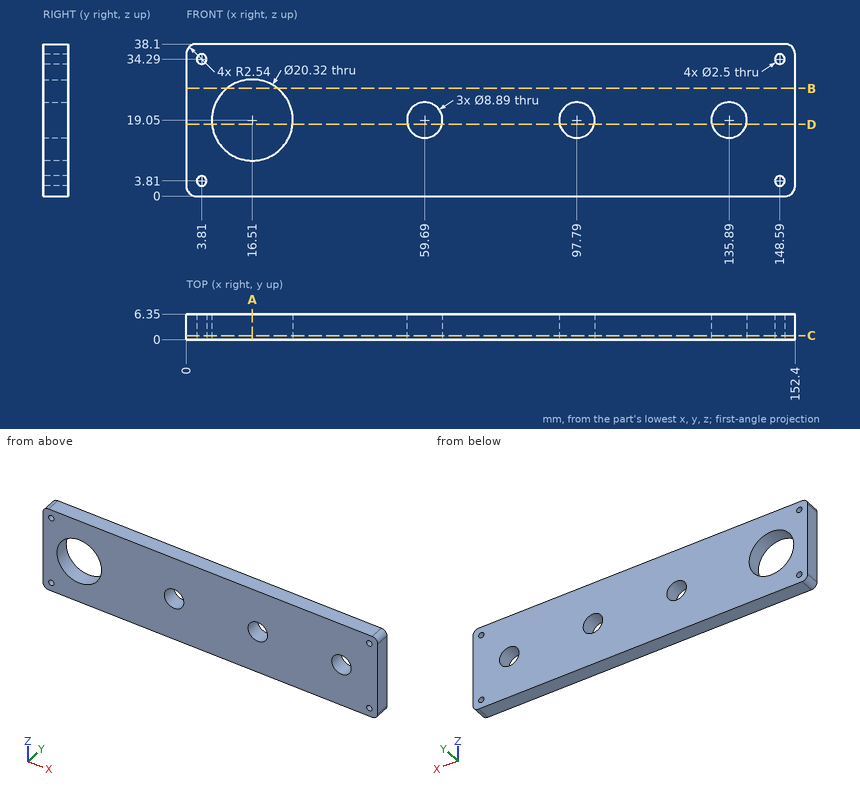
Could you check a few things on this drawing? It's one solid part, dimensions in mm from its lowest x, y, z. Coordinates: 2 decimals unless noted, no trailing zeros. Order: outer loops, then holes, each group sorted by start corner. A loop starts at its lowest first (then second) coordinate and runs counter-clockwise, first axis right, second up. Notation, with made-up numbers: M 17.5,80 L 68.5,80 A15 cw 68.5,95 Z; hole C -9,15 d11. An arc over 180 degrees is marked long. Answer as a JSON object with one key per item and string values. Group by question number.
(1) I need wall thicknesses on probe 1 along Z at (x, y) = (3.81, 3.5); probe 2 along X at (y, z) = (3.5, 19.05) (3 decimals); probe 3 along Z at (x, y) = (59.69, 4.5) (3 decimals). Which ranges of each line are inside material? Lowest first, please.
(2) Suppose I cut it at C-C, the plane y = 1. State how many separate pieces and enclosed holes the cut face has, then the cut area to 3 significant figures.
(3) Suppose I cut it at B-B, the plane z = 27. Please give me the cut outline in (x, y), then the cut area to 3 significant figures.
(4) Suppose I cut it at D-D, the plane z = 18. Please give me the cut outline in (x, y).
(5) Suppose I cut it at A-A, the plane x = 16.51. Please give me the cut outline in (y, z).
Values found:
{
 "1": {"probe 1": "z = 0 to 2.56, 5.06 to 33.04, 35.54 to 38.1", "probe 2": "x = 0 to 6.35, 26.67 to 55.245, 64.135 to 93.345, 102.235 to 131.445, 140.335 to 152.4", "probe 3": "z = 0 to 14.605, 23.495 to 38.1"},
 "2": {"separate pieces": "1", "enclosed holes": "8", "area": "5,270 mm^2"},
 "3": {"outline": "M 0,0 L 10.18,0 L 10.18,6.35 L 0,6.35 Z; M 22.84,0 L 152.4,0 L 152.4,6.35 L 22.84,6.35 Z", "area": "887 mm^2"},
 "4": {"outline": "M 0,0 L 6.4,0 L 6.4,6.35 L 0,6.35 Z; M 26.62,0 L 55.37,0 L 55.37,6.35 L 26.62,6.35 Z; M 64.01,0 L 93.47,0 L 93.47,6.35 L 64.01,6.35 Z; M 102.11,0 L 131.57,0 L 131.57,6.35 L 102.11,6.35 Z; M 140.21,0 L 152.4,0 L 152.4,6.35 L 140.21,6.35 Z"},
 "5": {"outline": "M 0,0 L 6.35,0 L 6.35,8.89 L 0,8.89 Z; M 0,29.21 L 6.35,29.21 L 6.35,38.1 L 0,38.1 Z"}
}
